Part print with two shaded views. Sizes in mm from the minimum x, y, z corner. Round coordinates to 2 decimals unless told otherwise and drop trailing zeros. Order: outer loops, then holes, each group sorted by start corner. A loop starts at its lowest first (then second) coordinate and runs counter-clockwise, first axis right, second up. Notation, with made-up numbers: M 77.25,85 L 94.25,85 A15 ccw 94.25,92 Z; hole C 87,61.5 d1. An arc over 180 degrees is marked long. Return JSON: item names as keys, results as strings. Group by question number.
Item 1: Slice it at B-B on y = 23.5. Write the cut outline in (x, z), then the cut area to 3 significant figures.
Item 2: Pull direction Y, two halves, no side cores. Call the marked faces 1, 2 and 3: pulls with the +Y half, pulls with the -Y half, needs draft (parallel to the pull), parting line crosses it, or undercut.
Item 3: Slice it at C-C on z = 2.7. Write the cut outline in (x, y).
Item 4: Pin check, flat tips, straight feed: pin 1 Ø12 at (x, y) = (16, 18.5) entering from -Z; pin 2 Ø2 at (y, z) = (12.5, 1.5) entering from -X; pin 3 Ø0.5 at (x, z) = (13, 0.5) entering from -Y; pin 4 Ø0.9 at (x, z) = (18.5, 2.5) entering from -Y. Stop position of each tip, or through.
Item 5: Probe line 1 along X through (y, z) = (18, 1.2); line 2 along X through (y, z) = (13.5, 0.4); line 3 along Y through (x, z) = (16, 2.55). List the from-to ranges inside material, lowest first.
Item 6: Slice it at A-A on x = 24.5. Write the cut outline in (y, z).
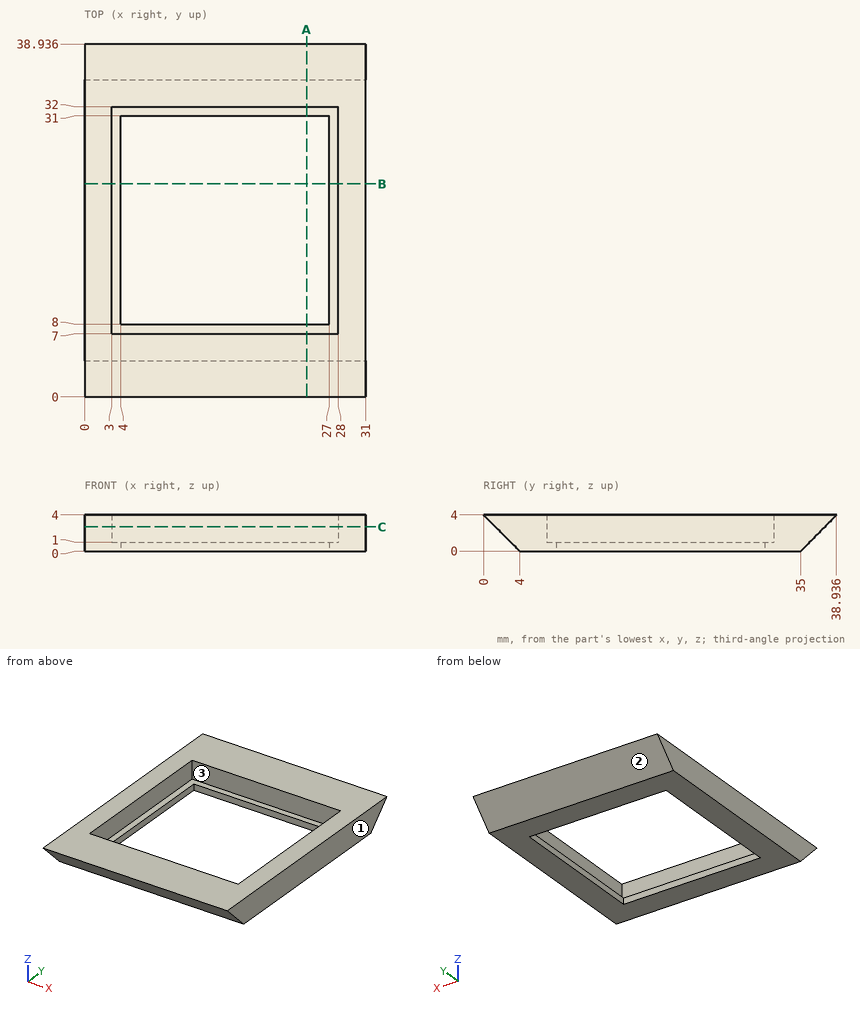
Output values:
{
 "1": {"outline": "M 0,0 L 4,0 L 4,1 L 3,1 L 3,4 L 0,4 Z; M 27,0 L 31,0 L 31,4 L 28,4 L 28,1 L 27,1 Z", "area": "26.0 mm²"},
 "2": {"face 1": "needs draft", "face 2": "pulls with the +Y half", "face 3": "undercut"},
 "3": {"outline": "M 0,1.3 L 31,1.3 L 31,37.66 L 0,37.66 Z; hole M 3,7 L 28,7 L 28,32 L 3,32 Z"},
 "4": {"pin 1": "through", "pin 2": "x = 0", "pin 3": "y = 3.25", "pin 4": "y = 1.05"},
 "5": {"line 1": "0 to 3, 28 to 31", "line 2": "0 to 4, 27 to 31", "line 3": "1.45 to 7, 32 to 37.51"},
 "6": {"outline": "M 0,4 L 4,0 L 8,0 L 8,1 L 7,1 L 7,4 Z; M 31,0 L 35,0 L 38.94,4 L 32,4 L 32,1 L 31,1 Z"}
}
